Geometry: see drawing. Coordinates: mm, zero at the bounding-box minimum. A direction names the side the tool comes from. Round coordinates to 2 decimals unless told otherwise and drop trailing zeros. Loops run counter-clockwise (first coordinate to the right, second up) from the corner with the lowest first, then second, coordinate; pieces in that order, holes last. Notation, with made-up numbers: M 17.5,-9.75 L 56.5,-9.75 A18 cw 56.5,1.25 Z; hole C 86,38 d9. An arc over 180 degrees is marked long. Answer as a JSON object with one key per item and string values.
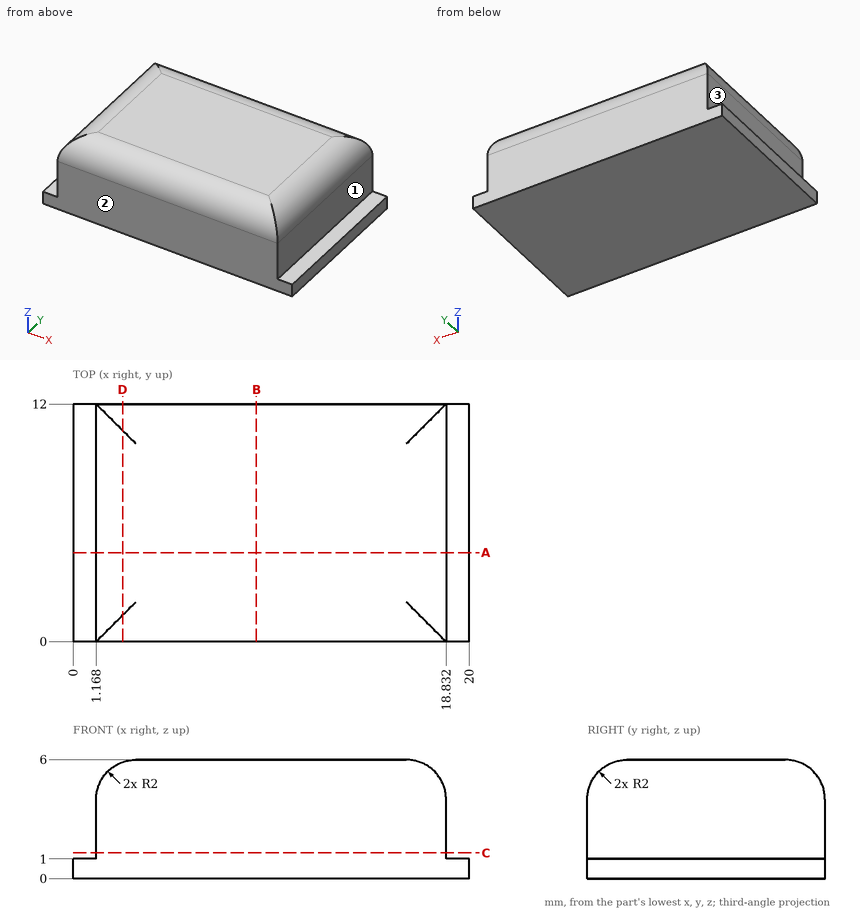
1) Ray query, line 1 (X direction, y = 1.25, z = 2.4); line 2 (Y direction, x = 10.75, z = 4.15) (1 decimal); line 3 (Z direction, x = 9.5, y = 1.25) (1 decimal). Return the intervals inside material, ascending.
Results:
{"line 1": "1.17 to 18.83", "line 2": "0 to 12", "line 3": "0 to 5.9"}
2) Section query B-B (x = 9.25). Return the cut outline in (y, z).
Results:
{"outline": "M 0,0 L 12,0 L 12,4 A2 ccw 10,6 L 2,6 A2 ccw 0,4 Z"}
3) Pin query (flat end, axial travel): P1, Ø1.5, axis at y = 4, z = 5.5, coming from the -X side; P2, Ø0.9, axis at y = 6.5, z = 2.5, coming from the -X side. Return the tip coordinate at first contact, or that it passes through.
Results:
{"P1": "x = 1.31", "P2": "x = 1.17"}
4) Section query D-D (x = 2.5). Return the cut outline in (y, z) (1 decimal).
Results:
{"outline": "M 0,0 L 12,0 L 12,4 A2 ccw 10.7,5.9 L 1.3,5.9 A2 ccw 0,4 Z"}
5) Section query C-C (z = 1.3). Return the cut outline in (x, y).
Results:
{"outline": "M 1.17,0 L 18.83,0 L 18.83,12 L 1.17,12 Z"}
6) Reachability of the marked faces 1, 2 and 3 from +Z, -Z, +X, -X, +Y, -Y: full face, straight path, thin tool, end or side. Return the list, or none.
Results:
{"face 1": "+Z, +X, +Y, -Y", "face 2": "+Z, -Z, +X, -X, -Y", "face 3": "+Z, -X, +Y, -Y"}
7) Section query A-A (y = 4.5). Return the cut outline in (x, z).
Results:
{"outline": "M 0,0 L 20,0 L 20,1 L 18.83,1 L 18.83,4 A2 ccw 16.83,6 L 3.17,6 A2 ccw 1.17,4 L 1.17,1 L 0,1 Z"}
